Geometry: final body of the model. Coordinates: model frame, mm. Face numbers are marked on the shaded views. A direction names the side the tool comes from. Give positions to 0.01 mm unless a question says otherwise; leave off trailing zeros. Loops run counter-clockwise (first coordinate to the right, second up) from the corner with the lowest first, then second, coordinate; pieces in that order, holes last. Notation, with made-up numbers: (-10, 44.25) - (-6, 44.25) arc R27 ccw to (-6, 65.25) - close; hole circle Ø3 at (18.25, 71). An arc over 180 degrees is marked (long way). Use one line per item in the form item = value.
```python
from build123d import *

# Parameters (mm, degrees)
SKETCH1_R           = 12.5
SKETCH1_R_2         = 3.25
BOSS_EXTRUDE1_DEPTH = 10
CUT_EXTRUDE1_REACH  = 27
SKETCH2_R           = 4.95
BOSS_EXTRUDE2_DEPTH = 0.95


with BuildPart() as part:
    # Sketch1 → Boss-Extrude1 (new body)
    with BuildSketch(Plane(origin=(0, 0, 0), x_dir=(1, 0, 0), z_dir=(0, 1, 0))):
        with BuildLine():
            ThreePointArc((12.5, 15), (0, 2.5), (-12.5, 15))
            Line((-12.5, 15), (-12.5, -14.999999966))
            ThreePointArc((-12.5, -14.999999966), (1.7e-08, -2.5), (12.5, -15))
            Line((12.5, -15), (12.5, 15))
        make_face()
        with Locations((0, 15)):
            Circle(SKETCH1_R)
        with Locations((0, 15)):
            Circle(SKETCH1_R_2, mode=Mode.SUBTRACT)
        with Locations((0, -15)):
            Circle(SKETCH1_R)
        with Locations((0, -15)):
            Circle(SKETCH1_R_2, mode=Mode.SUBTRACT)
    extrude(amount=BOSS_EXTRUDE1_DEPTH)

    # Sketch2 → Cut-Extrude1 (cut, up to next)
    with BuildSketch(Plane(origin=(12.5, 0, 0), x_dir=(0, 0, -1), z_dir=(1, 0, 0)), mode=Mode.PRIVATE) as cut_extrude1_sk1:
        with Locations((0, 10)):
            Circle(SKETCH2_R)
    cut_extrude1_tool1 = extrude(cut_extrude1_sk1.sketch, amount=-CUT_EXTRUDE1_REACH, mode=Mode.PRIVATE) & part.part
    add(cut_extrude1_tool1.solids().sort_by_distance((12.5, 10, 0))[0], mode=Mode.SUBTRACT)

    # Sketch3 → Boss-Extrude2 (add, symmetric)
    with BuildSketch(Plane(origin=(0, 0, 0), x_dir=(0, 0, -1), z_dir=(1, 0, 0))):
        with BuildLine():
            Line((4.95, 10), (4.5, 10))
            ThreePointArc((4.5, 10), (0, 5.5), (-4.5, 10))
            Line((-4.5, 10), (-4.95, 10))
            ThreePointArc((-4.95, 10), (0, 5.05), (4.95, 10))
        make_face()
    extrude(amount=BOSS_EXTRUDE2_DEPTH, both=True)


solid = part.part
```
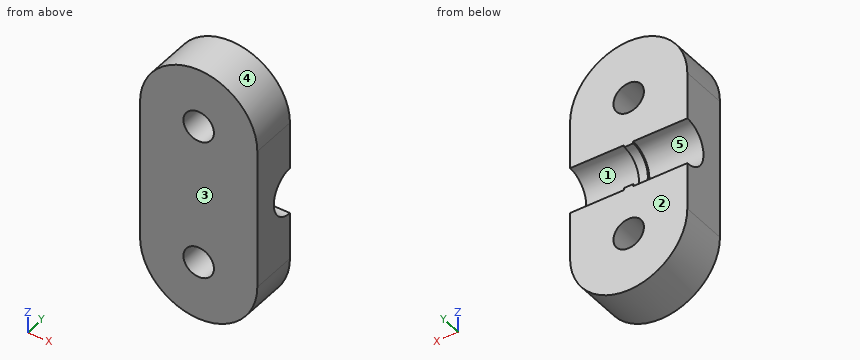
(1) Cut plane D-D (y = 4.25). Return the cut outline in (x, z).
Solution:
outline = (-12.5, -15) arc R12.5 ccw to (12.5, -15) - (12.5, 15) arc R12.5 ccw to (-12.5, 15) - close; hole circle Ø6.5 at (0, -15); hole circle Ø6.5 at (0, 15)
(2) Cut plane C-C (x = 0). Return the cut outline in (y, z).
Solution:
outline = (0, -27.5) - (10, -27.5) - (10, -18.25) - (0, -18.25) - close; (0, -11.75) - (10, -11.75) - (10, -4.5) arc R4.5 cw to (10, 4.5) - (10, 11.75) - (0, 11.75) - close; (0, 18.25) - (10, 18.25) - (10, 27.5) - (0, 27.5) - close
(3) Pull-direction query (Z, two-part tool) for the marked faces 3, 4 and 5; classes: released by +Z, released by -Z, zero draft, split by the parting line, or undercut.
Solution:
face_3 = zero draft
face_4 = released by +Z
face_5 = undercut
(4) Pin query (flat end, axial travel): P1, Ø4, axis at x = 5, y = 1.5, coming from the +Z side; P2, Ø4, axis at x = -2.5, z = -14.5, coming from the -Y side. Return the tip coordinate at first contact, or that it passes through.
Solution:
P1 = 27.13
P2 = 0
(5) Cut plane B-B (z = 0). Return the cut outline in (x, y), plus the area to 3 significant figures.
Solution:
outline = (-12.5, 0) - (12.5, 0) - (12.5, 5.05) - (0.95, 5.05) - (0.95, 5.5) - (-0.95, 5.5) - (-0.95, 5.05) - (-12.5, 5.05) - close
area = 127 mm2
(6) Material intervals for L1, parallel to Z at x = 0, y = 5; L2, parallel to X at y = 2.5, z = -15; L3, parallel to Z at x = -2.75, y = 5.5, sorted ascending. Write a range as from..to.
Solution:
L1 = -27.5..-18.25, -11.75..11.75, 18.25..27.5
L2 = -12.5..-3.25, 3.25..12.5
L3 = -27.19..-16.73, -13.27..-2.06, 2.06..13.27, 16.73..27.19
(7) Access query for the marked faces 1 and 2. Directions: +Z, -Z, +X, -X, +Y, -Y. A direction counts if a zero-diameter tool reaches every point of the face in a straight line with its end or side. Return the directions, or none.
Solution:
face_1 = +X, +Y
face_2 = +Z, -Z, +X, -X, +Y
(8) Cut plane A-A (y = 8). Return the cut outline in (x, z), plus the area to 3 significant figures.
Solution:
outline = (-12.5, -15) arc R12.5 ccw to (12.5, -15) - (12.5, -4.53) - (0.95, -4.53) - (0.95, -4.03) - (-0.95, -4.03) - (-0.95, -4.53) - (-12.5, -4.53) - close; (-12.5, 4.53) - (-0.95, 4.53) - (-0.95, 4.03) - (0.95, 4.03) - (0.95, 4.53) - (12.5, 4.53) - (12.5, 15) arc R12.5 ccw to (-12.5, 15) - close; hole circle Ø6.5 at (0, -15); hole circle Ø6.5 at (0, 15)
area = 950 mm2
